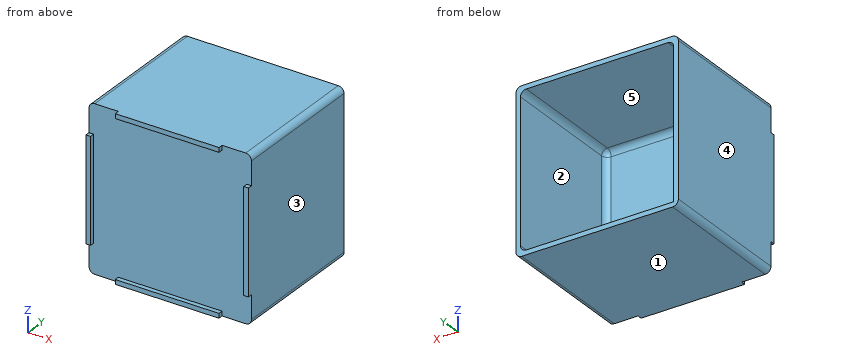
Autodesk Inventor part; units mm, degrees
ref_plane "YZ Plane" through (0, 0, 0) normal (1, 0, 0) x (0, 1, 0)
ref_plane "XZ Plane" through (0, 0, 0) normal (0, 1, 0) x (-1, 0, 0)
ref_plane "XY Plane" through (0, 0, 0) normal (0, 0, 1) x (1, 0, 0)
sketch "Эскиз1" plane through (0, 0, 0) normal (0, 1, 0) x (-1, 0, 0)
  line L0 (-70.5, 70.5) -> (70.5, 70.5)
  line L1 (70.5, 70.5) -> (70.5, -70.5)
  line L2 (70.5, -70.5) -> (-70.5, -70.5)
  line L3 (-70.5, -70.5) -> (-70.5, 70.5)
  line L4 (-70.5, 70.5) -> (70.5, -70.5) construction
  line L5 (70.5, 70.5) -> (-70.5, -70.5) construction
  point P0 (0, 0)
  dimension "d0" = 141
extrude "Выдавливание1" add sketch "Эскиз1" along normal blind 120
sketch "Эскиз2" plane through (0, 120, 0) normal (0, 1, 0) x (1, 0, 0)
  line L0 (66.5, -66.5) -> (-66.5, -66.5)
  line L1 (-66.5, -66.5) -> (-66.5, 66.5)
  line L2 (-66.5, 66.5) -> (66.5, 66.5)
  line L3 (66.5, 66.5) -> (66.5, -66.5)
  line L4 (66.5, -66.5) -> (-66.5, 66.5) construction
  line L5 (-66.5, -66.5) -> (66.5, 66.5) construction
  line L6 (-70.5, 70.5) -> (-70.5, -70.5)
  point P0 (0, 0)
  dimension "d3" = 4
extrude "Выдавливание2" cut sketch "Эскиз2" against normal blind 110
fillet "Сопряжение1" radius 5 11 edges at (70.5, 60, 70.5) (66.5, 65, 66.5) (70.5, 60, -70.5) (66.5, 65, -66.5) (-66.5, 65, 66.5) (-66.5, 10, 0) (0, 10, 66.5) (66.5, 10, 0) (0, 10, -66.5) (-70.5, 60, -70.5) (-70.5, 60, 70.5)
sketch "Эскиз3" plane through (0, 0, 0) normal (0, -1, 0) x (1, 0, 0)
  arc A0 (-65.5, 70.5) -> (-70.5, 65.5) centre (-65.5, 65.5) ccw
  line L0 (-70.5, -65.5) -> (-70.5, 65.5)
  arc A1 (-70.5, -65.5) -> (-65.5, -70.5) centre (-65.5, -65.5) ccw
  line L1 (65.5, -70.5) -> (-65.5, -70.5)
  arc A2 (65.5, -70.5) -> (70.5, -65.5) centre (65.5, -65.5) ccw
  line L2 (70.5, 65.5) -> (70.5, -65.5)
  arc A3 (70.5, 65.5) -> (65.5, 70.5) centre (65.5, 65.5) ccw
  line L3 (-65.5, 70.5) -> (65.5, 70.5)
  line L4 (45, -70.5) -> (-45, -70.5)
  line L5 (-45, -70.5) -> (-45, -66.5)
  line L6 (-45, -66.5) -> (45, -66.5)
  line L7 (45, -66.5) -> (45, -70.5)
  line L8 (70.5, 65.5) -> (70.5, -65.5)
  line L9 (70.5, -45) -> (70.5, 45)
  line L10 (70.5, 45) -> (66.5, 45)
  line L11 (66.5, 45) -> (66.5, -45)
  line L12 (66.5, -45) -> (70.5, -45)
  line L13 (-70.5, -45) -> (-70.5, 45)
  line L14 (-70.5, 45) -> (-66.5, 45)
  line L15 (-66.5, 45) -> (-66.5, -45)
  line L16 (-66.5, -45) -> (-70.5, -45)
  line L17 (-65.5, 70.5) -> (65.5, 70.5)
  line L18 (45, 70.5) -> (-45, 70.5)
  line L19 (-45, 70.5) -> (-45, 66.5)
  line L20 (-45, 66.5) -> (45, 66.5)
  line L21 (45, 66.5) -> (45, 70.5)
  line L22 (0, 0) -> (0, -15.64) construction
  line L23 (0, 0) -> (-17.2484, 0) construction
  point P0 (45, 70.5)
  point P1 (-45, 70.5)
  point P2 (70.5, 45)
  dimension "d7" = 4
  dimension "d8" = 90
extrude "Выдавливание3" add sketch "Эскиз3" along normal blind 4 contours L3 L21 L20 L19 | L14 L15 L16 L0 | L2 L12 L11 L10 | L5 L6 L7 L1
properties part number "сосуд"
Check sheet for the modelled part. Datum: model origin and axes. Units: mm. Face numbers are marked on the shaded views. A direction names the side the tool comes from. Give positions to 0.01 mm unless a question says otherwise; leave off trailing zeros. Write each loop counter-clockwise with the first axis right and the second up, starting at its lowest first coordinate (ties: lowest second). Pieces come first, ordered by that corner, then holes.
Item 1: Access from +Z, -Z, +X, -X, +Y, -Y to the whole of each face (thin tool, end or side, straight path). Record for the marked faces 4 and 5.
Item 2: Scan lines: L1, parallel to X at y = 95, z = 32.5; L2, parallel to Y at x = -52, z = -54. Record each from-to range of solid material in increasing order.
Item 3: Cross-section at C-C (z = -30.5). Enter the section's corners in (x, y), and give its area (3 significant figures).
Item 4: Gauge pin test, flat ends, axial feed: pin 1 (4 mm diameter, centred on x = 37, z = 18.5, fed in from -Y); pin 2 (4.5 mm diameter, centred on x = -68.5, y = -1.5, fed in from +Z); pin 3 (2 mm diameter, centred on x = -69, y = -3, fed in from -Z). Record the tip position at first contact, or that the pin passes through.
Item 5: Cross-section at B-B (x = -6). Enter the section's corners in (y, z).
Item 6: Cross-section at D-D (x = 58). Enter the section's corners in (y, z).
Item 7: Cross-section at A-A (y = 26). Enter the section's corners in (x, z).
Item 8: Draft check along X on the marked faces 1, 2 and 3. Enter one of: released by +X, released by -X, zero draft, split by the parting line, or undercut.
Report:
1. face 4: +Z, -Z, -X, +Y, -Y
1. face 5: +Y
2. L1: x = -70.5 to -66.5, 66.5 to 70.5
2. L2: y = 0 to 10
3. outline: (-70.5, -4) - (-66.5, -4) - (-66.5, 0) - (66.5, 0) - (66.5, -4) - (70.5, -4) - (70.5, 120) - (66.5, 120) - (66.5, 15) arc R5 cw to (61.5, 10) - (-61.5, 10) arc R5 cw to (-66.5, 15) - (-66.5, 120) - (-70.5, 120) - close
3. area: 2,330 mm2
4. pin 1: stops at y = 0
4. pin 2: stops at z = 70.32
4. pin 3: stops at z = -45
5. outline: (-4, -70.5) - (120, -70.5) - (120, -66.5) - (15, -66.5) arc R5 cw to (10, -61.5) - (10, 61.5) arc R5 cw to (15, 66.5) - (120, 66.5) - (120, 70.5) - (-4, 70.5) - (-4, 66.5) - (0, 66.5) - (0, -66.5) - (-4, -66.5) - close
6. outline: (0, -70.5) - (120, -70.5) - (120, -66.5) - (15, -66.5) arc R5 cw to (10, -61.5) - (10, 61.5) arc R5 cw to (15, 66.5) - (120, 66.5) - (120, 70.5) - (0, 70.5) - close
7. outline: (-70.5, -65.5) arc R5 ccw to (-65.5, -70.5) - (65.5, -70.5) arc R5 ccw to (70.5, -65.5) - (70.5, 65.5) arc R5 ccw to (65.5, 70.5) - (-65.5, 70.5) arc R5 ccw to (-70.5, 65.5) - close; hole (-66.5, -66.5) - (61.5, -66.5) arc R5 ccw to (66.5, -61.5) - (66.5, 61.5) arc R5 ccw to (61.5, 66.5) - (-61.5, 66.5) arc R5 ccw to (-66.5, 61.5) - close
8. face 1: zero draft
8. face 2: undercut
8. face 3: released by +X
